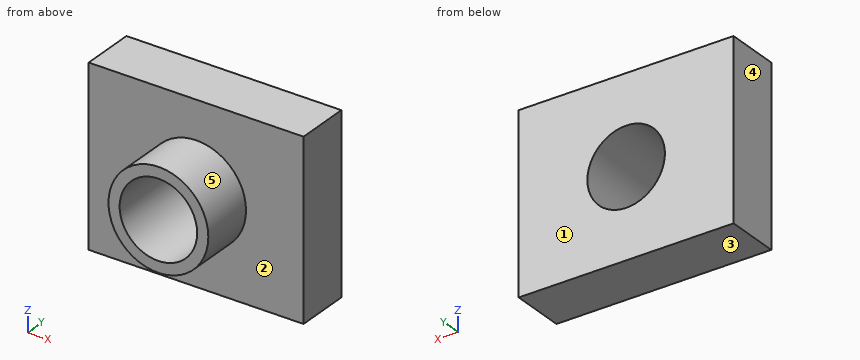
```python
from build123d import *

# Parameters (mm, degrees)
F0_W     = 101.3161987066
F0_H     = 83.1388831139
F1_DEPTH = 25.4
F2_R     = 18.2729381932
F3_DEPTH = 25.4
F4_R     = 23.5410292958
F4_R_2   = 18.2729381932
F5_DEPTH = 25.4


with BuildPart() as f1:
    # F0 (on Front) → F1 (new body)
    with BuildSketch(Plane.XZ):
        Rectangle(F0_W, F0_H)
    extrude(amount=F1_DEPTH)

    # F2 (on face) → F3 (cut)
    with BuildSketch(Plane.XZ.offset(25.4)):
        Circle(F2_R)
    extrude(amount=-F3_DEPTH, mode=Mode.SUBTRACT)

    # F4 (on face) → F5 (join)
    with BuildSketch(Plane.XZ.offset(25.4)):
        Circle(F4_R)
        Circle(F4_R_2, mode=Mode.SUBTRACT)
    extrude(amount=F5_DEPTH)


solid = f1.part
```
The model under review builds one solid part; all positions refer to its coordinate system, in mm. Face numbers are marked on the shaded views. A direction names the side the tool comes from. Round coordinates to 2 decimals unless told otherwise and drop trailing zeros. Loops run counter-clockwise (first coordinate to the right, second up) from the corner with the lowest first, then second, coordinate; pieces in that order, holes last. Notation, with made-up numbers: M 57.25,-31 L 96.25,-31 A29 ccw 96.25,-8 Z; hole C 25,-34 d7. An arc over 180 degrees is marked long. Write item = value, one per line.
Item 1: The part is to be moulded in two halves that separate along Y. For the marked faces 1, 2 and 3, say which applies: released by +Y, released by -Y, zero draft, split by the parting line, or undercut.
Return value:
face_1 = released by +Y
face_2 = released by -Y
face_3 = zero draft
Item 2: Take a section at B-B on z = 0. Write out the cut boundary in (x, y), then the cut area to 3 significant figures.
Return value:
outline = M -50.66,-25.4 L -23.54,-25.4 L -23.54,-50.8 L -18.27,-50.8 L -18.27,0 L -50.66,0 Z; M 18.27,-50.8 L 23.54,-50.8 L 23.54,-25.4 L 50.66,-25.4 L 50.66,0 L 18.27,0 Z
area = 1,910 mm2
Item 3: Take a section at D-D on z = 32. Write out the cut boundary in (x, y).
Return value:
outline = M -50.66,-25.4 L 50.66,-25.4 L 50.66,0 L -50.66,0 Z
Item 4: Machinability: for the marked faces 4 and 5, which of the approach directions +Z, -Z, +X, -X, +Y, -Y give a long, thin tool a straight path to every point of the face, cutting with its end or side? Answer none if there is none.
Return value:
face_4 = +Z, -Z, -X, +Y, -Y
face_5 = -Y
Item 5: For line 1 (Z direction, x = 0, y = -24); line 2 (X direction, y = -38, z = -0.5), list the stretches that pass through material, from the lowest coordinate up. Write a range as [from, to].
Return value:
line_1 = [-41.57, -18.27], [18.27, 41.57]
line_2 = [-23.54, -18.27], [18.27, 23.54]
Item 6: Take a section at A-A on x = 0. Write out the cut boundary in (y, z).
Return value:
outline = M -50.8,-23.54 L -25.4,-23.54 L -25.4,-41.57 L 0,-41.57 L 0,-18.27 L -50.8,-18.27 Z; M -50.8,18.27 L 0,18.27 L 0,41.57 L -25.4,41.57 L -25.4,23.54 L -50.8,23.54 Z
Item 7: Insertion check: P1, Ø1, axis at y = -36.5, z = 5, coming from the -X side; P2, Ø22, axis at x = 0, z = 0, coming from the -Y side; P3, Ø6, axis at y = -33.5, z = 12, coming from the +X side. Each pin has a flat end and moves straight along its axis. Give the tip position at first contact, or say it passes through.
Return value:
P1 = -23.11
P2 = through
P3 = 21.75
Item 8: Take a section at C-C on y = -11. Write out the cut boundary in (x, z), then the cut area to 3 significant figures.
Return value:
outline = M -50.66,-41.57 L 50.66,-41.57 L 50.66,41.57 L -50.66,41.57 Z; hole C 0,0 d36.55
area = 7,370 mm2
